The figure shows three views and two pictorial views of one solid part (mm, origin at its lowest corner). Answer the questions. Round coordinates to 2 decimals unless told otherwise and drop trailing zeros. Order: outer loops, then holes, each group sorted by start corner. A loop starts at its lowest first (then second) coordinate and runs counter-clockwise, first axis right, second up. Notation, with made-up numbers: (52.5, 30) - (58.5, 30) arc R24 ccw to (58.5, 68) - close; hole circle Ø4 at (77.25, 12.5). An arc over 180 degrees is marked (long way). Answer in a Markdown table with one row per item.
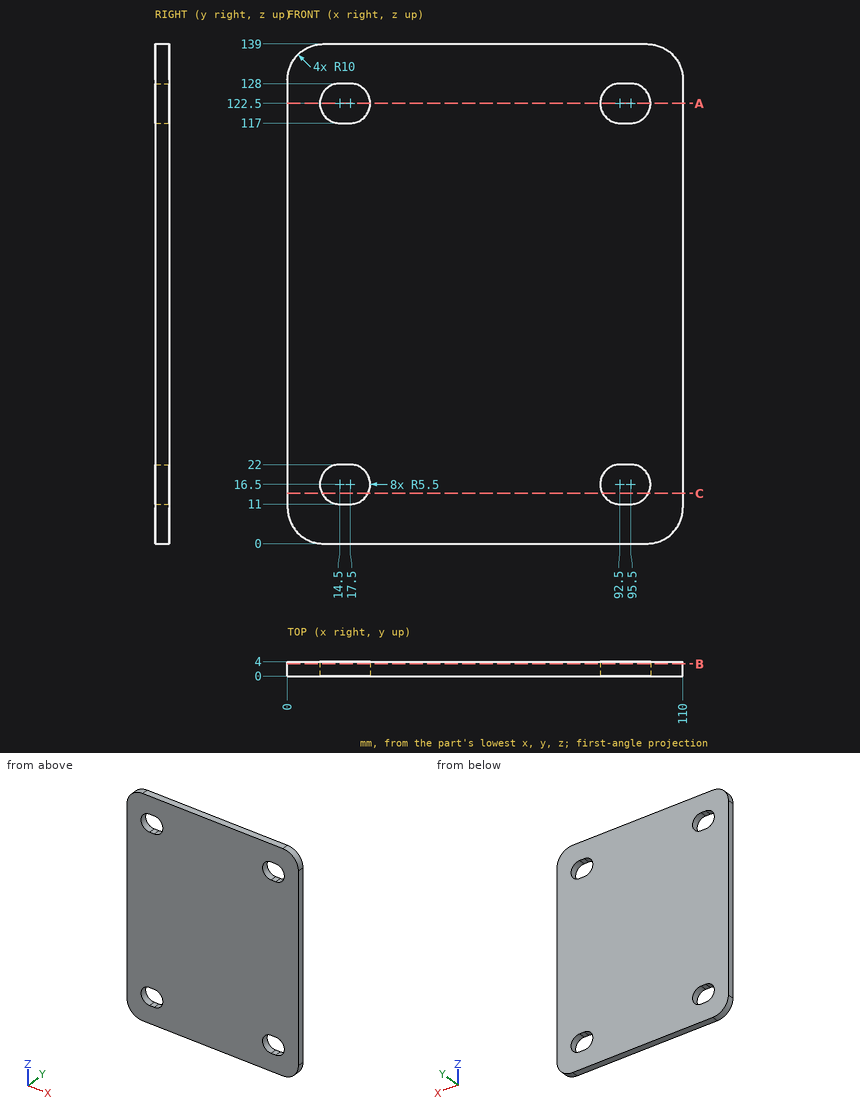
1) Find section A-A, the plane z = 122.5. Give the vertices of the cut face in (x, y), then the cut area to 3 significant figures.
Filled in:
| item | result |
|---|---|
| outline | (0, 0) - (9, 0) - (9, 4) - (0, 4) - close; (23, 0) - (87, 0) - (87, 4) - (23, 4) - close; (101, 0) - (110, 0) - (110, 4) - (101, 4) - close |
| area | 328 mm^2 |
2) Find section B-B, the plane y = 3.4. Give the vertices of the cut face in (x, z), then the cut area to 3 significant figures.
Filled in:
| item | result |
|---|---|
| outline | (0, 10) arc R10 ccw to (10, 0) - (100, 0) arc R10 ccw to (110, 10) - (110, 129) arc R10 ccw to (100, 139) - (10, 139) arc R10 ccw to (0, 129) - close; hole (14.5, 11) - (17.5, 11) arc R5.5 ccw to (17.5, 22) - (14.5, 22) arc R5.5 ccw to start; hole (14.5, 117) - (17.5, 117) arc R5.5 ccw to (17.5, 128) - (14.5, 128) arc R5.5 ccw to start; hole (92.5, 11) - (95.5, 11) arc R5.5 ccw to (95.5, 22) - (92.5, 22) arc R5.5 ccw to start; hole (92.5, 117) - (95.5, 117) arc R5.5 ccw to (95.5, 128) - (92.5, 128) arc R5.5 ccw to start |
| area | 14,700 mm^2 |
3) Find the intervals of material crossed by probe 1 along Z at (x, y) = (92.5, 2.2); probe 2 along X at (y, z) = (2.5, 122); probe 3 along Z at (x, y) = (99, 3.45), in increasing order. Write a range as from..to.
Filled in:
| item | result |
|---|---|
| probe 1 | z = 0..11, 22..117, 128..139 |
| probe 2 | x = 0..9.02, 22.98..87.02, 100.98..110 |
| probe 3 | z = 0..12.26, 20.74..118.26, 126.74..139 |
4) Find section C-C, the plane z = 14. Give the vertices of the cut face in (x, y).
Filled in:
| item | result |
|---|---|
| outline | (0, 0) - (9.6, 0) - (9.6, 4) - (0, 4) - close; (22.4, 0) - (87.6, 0) - (87.6, 4) - (22.4, 4) - close; (100.4, 0) - (110, 0) - (110, 4) - (100.4, 4) - close |
